Design review of the part built by this model. Coordinates are the model's own, in mm. A direction names the side the tool comes from. Round coordinates to 2 decimals unless told otherwise and drop trailing zeros. Loops run counter-clockwise (first coordinate to the right, second up) from the corner with the lowest first, then second, coordinate; pieces in that order, holes last. Notation, with made-up numbers: (55.5, 52) - (94.5, 52) arc R12 cw to (94.5, 75) - close; hole circle Ø2 at (8.5, 83.5). An arc over 180 degrees is marked (long way). Return JSON: item names as keys, results as strings. Group by question number.
from build123d import *

# Parameters (mm, degrees)
BOSS_EXTRUDE1_DEPTH     = 3
SKETCH3_W               = 5
SKETCH3_H               = 6.177085
CUT_EXTRUDE1_DEPTH      = 1
CUT_EXTRUDE1_DEPTH_BACK = 4


with BuildPart() as part:
    # Sketch2 → Boss-Extrude1 (new body)
    with BuildSketch(Plane(origin=(0, 0, 0), x_dir=(1, 0, 0), z_dir=(0, 1, 0))):
        Polygon((-6.5, -81.77085), (-6.5, -98.12502), (6.5, -98.12502), (6.5, -81.77085), (9.5, -81.77085), (9.5, -65.41668), (6.5, -65.41668), (6.5, -49.06251), (9.5, -49.06251), (9.5, -32.70834), (6.5, -32.70834), (6.5, -16.35417), (9.5, -16.35417), (9.5, 0), (6.5, 0), (6.5, 16.35417), (9.5, 16.35417), (9.5, 32.70834), (6.5, 32.70834), (6.5, 49.06251), (9.5, 49.06251), (9.5, 65.41668), (6.5, 65.41668), (-6.5, 65.41668), (-9.5, 65.41668), (-9.5, 49.06251), (-6.5, 49.06251), (-6.5, 32.70834), (-9.5, 32.70834), (-9.5, 16.35417), (-6.5, 16.35417), (-6.5, 0), (-9.5, 0), (-9.5, -16.35417), (-6.5, -16.35417), (-6.5, -32.70834), (-9.5, -32.70834), (-9.5, -49.06251), (-6.5, -49.06251), (-6.5, -65.41668), (-9.5, -65.41668), (-9.5, -81.77085), align=None)
    extrude(amount=BOSS_EXTRUDE1_DEPTH)

    # Sketch3 → Cut-Extrude1 (cut, two sides)
    with BuildSketch(Plane(origin=(0, 3, 0), x_dir=(1, 0, 0), z_dir=(0, 1, 0))) as cut_extrude1_sk:
        Polygon((-5.5, 53.06251), (-5.5, 61.41668), (5.5, 61.41668), (5.5, 53.06251), (2.5, 53.06251), (2.5, 44.885425), (-2.5, 44.885425), (-2.5, 53.06251), align=None)
        Polygon((-2.5, 28.70834), (-2.5, 36.885425), (2.5, 36.885425), (2.5, 28.70834), (5.5, 28.70834), (5.5, 20.35417), (2.5, 20.35417), (2.5, 12.177085), (-2.5, 12.177085), (-2.5, 20.35417), (-5.5, 20.35417), (-5.5, 28.70834), align=None)
        Polygon((-5.5, -4), (-2.5, -4), (-2.5, 4.177085), (2.5, 4.177085), (2.5, -4), (5.5, -4), (5.5, -12.35417), (2.5, -12.35417), (2.5, -20.531255), (-2.5, -20.531255), (-2.5, -12.35417), (-5.5, -12.35417), align=None)
        Polygon((-5.5, -69.41668), (-2.5, -69.41668), (-2.5, -61.239595), (2.5, -61.239595), (2.5, -69.41668), (5.5, -69.41668), (5.5, -77.77085), (2.5, -77.77085), (2.5, -85.947935), (-2.5, -85.947935), (-2.5, -77.77085), (-5.5, -77.77085), align=None)
        with Locations((0, -89.0364775)):
            Rectangle(SKETCH3_W, SKETCH3_H)
        Polygon((-5.5, -36.70834), (-2.5, -36.70834), (-2.5, -28.531255), (2.5, -28.531255), (2.5, -36.70834), (5.5, -36.70834), (5.5, -45.06251), (2.5, -45.06251), (2.5, -53.239595), (-2.5, -53.239595), (-2.5, -45.06251), (-5.5, -45.06251), align=None)
    extrude(amount=CUT_EXTRUDE1_DEPTH, mode=Mode.SUBTRACT)
    extrude(cut_extrude1_sk.sketch, amount=-CUT_EXTRUDE1_DEPTH_BACK, mode=Mode.SUBTRACT)


solid = part.part
Q1. Draft analysis for pull direction X (two halves, no side actions). For faces 6 (the flat face through (-9.5, 1, -57)), 7 (the flat face through (0, 1, 98.125)), 8 (the flat face through (5.5, 2, 74)), 9 (the flat face through (-2.5, 2, 33)), state which applies: pulls with the +X half, pulls with the -X half, needs draft (parallel to the pull), parting line crosses it, or undercut.
Q2. Add section A-A, the plane x = 0.25. State the section outline as (y, z) points, plus the area to 3 significant figures.
Q3. Insertion check: pin 1 Ø0.9 at (y, z) = (1.5, 61) entering from -X; pin 2 Ø0.9 at (x, y) = (8.5, 1.5) entering from +Z. Each pin has a flat end and moves straight along its axis. Give the tip position at first contact, or say it passes through.
Q4. Add section C-C, the plane x = -8. State the section outline as (y, z) points.
Q5. Tool access review of faces 1 (the flat face through (-6.5, 1, 90)), 2 (the flat face through (-2.5, 2, 49)), 3 (the flat face through (-6.5, 1, -8)), 4 (the flat face through (6.5, 1, -41)), 5 (the flat face through (9.5, 1, 74)): name each direction out of +Z, -Z, +X, -X, +Y, -Y from which nothing blocks a thin tool from reaching the whole face with its end or side.
Q6. Add section B-B, the plane z = -54.5. State the section outline as (x, y) points.
Q7. Add section D-D, the plane y = 0.75. Give the number of separate pieces and of enclosed holes in the cut face, plus the area to 3 significant figures.
Q8. For line 1 (Z direction, x = -8.5, y = 0.8); line 2 (Z direction, x = -3, y = 1.7); line 3 (Z direction, x = -1.5, y = 2.45), list the stretches that pass through material, from the lowest coordinate up.
Evaluation:
{
 "1": {"face 6": "pulls with the -X half", "face 7": "needs draft", "face 8": "undercut", "face 9": "undercut"},
 "2": {"outline": "(0, -65.42) - (3, -65.42) - (3, -61.42) - (0, -61.42) - close; (0, -44.89) - (3, -44.89) - (3, -36.89) - (0, -36.89) - close; (0, -12.18) - (3, -12.18) - (3, -4.18) - (0, -4.18) - close; (0, 20.53) - (3, 20.53) - (3, 28.53) - (0, 28.53) - close; (0, 53.24) - (3, 53.24) - (3, 61.24) - (0, 61.24) - close; (0, 92.13) - (3, 92.13) - (3, 98.13) - (0, 98.13) - close", "area": "126 mm²"},
 "3": {"pin 1": "x = -6.5", "pin 2": "z = 81.77"},
 "4": {"outline": "(0, -65.42) - (3, -65.42) - (3, -49.06) - (0, -49.06) - close; (0, -32.71) - (3, -32.71) - (3, -16.35) - (0, -16.35) - close; (0, 0) - (3, 0) - (3, 16.35) - (0, 16.35) - close; (0, 32.71) - (3, 32.71) - (3, 49.06) - (0, 49.06) - close; (0, 65.42) - (3, 65.42) - (3, 81.77) - (0, 81.77) - close"},
 "5": {"face 1": "+Z, -X, +Y, -Y", "face 2": "+Y, -Y", "face 3": "-X, +Y, -Y", "face 4": "+X, +Y, -Y", "face 5": "+Z, -Z, +X, +Y, -Y"},
 "6": {"outline": "(-9.5, 0) - (-5.5, 0) - (-5.5, 3) - (-9.5, 3) - close; (5.5, 0) - (9.5, 0) - (9.5, 3) - (5.5, 3) - close"},
 "7": {"separate pieces": "1", "enclosed holes": "5", "area": "1,760 mm²"},
 "8": {"line 1": "-65.42 to -49.06, -32.71 to -16.35, 0 to 16.35, 32.71 to 49.06, 65.42 to 81.77", "line 2": "-65.42 to -61.42, -53.06 to -28.71, -20.35 to 4, 12.35 to 36.71, 45.06 to 69.42, 77.77 to 98.13", "line 3": "-65.42 to -61.42, -44.89 to -36.89, -12.18 to -4.18, 20.53 to 28.53, 53.24 to 61.24, 92.13 to 98.13"}
}
